from build123d import *

# Parameters (mm, degrees)
ESQUISSE1_W                       = 180
ESQUISSE1_H                       = 330
BOSS_EXTRU_1_DEPTH                = 6
ESQUISSE2_R                       = 2
ESQUISSE2_R_2                     = 10
ESQUISSE2_R_3                     = 1.4
ESQUISSE2_W                       = 55
ESQUISSE2_H                       = 8
ESQUISSE2_H_2                     = 44
ENL_V_MAT_BLOC_MOTEUR_BILLE_DEPTH = 376.946804748
ESQUISSE3_W                       = 6
ESQUISSE3_H                       = 25
ESQUISSE3_W_2                     = 10
ESQUISSE3_H_2                     = 6
ESQUISSE3_W_3                     = 30
ESQUISSE3_H_3                     = 40
ENL_V_MAT_ENCOCHE_DEPTH           = 376.946804748


with BuildPart() as part:
    # Esquisse1 → Boss.-Extru.1 (new body)
    with BuildSketch(Plane.XY):
        with Locations((-90, 165)):
            Rectangle(ESQUISSE1_W, ESQUISSE1_H)
    extrude(amount=BOSS_EXTRU_1_DEPTH)

    # Esquisse2 → Enlèv. mat bloc moteur + bille (cut, through all)
    with BuildSketch(Plane.XY.offset(6)):
        with Locations((-176, 326)):
            Circle(ESQUISSE2_R)
        with Locations((-160, 305)):
            Circle(ESQUISSE2_R_2)
        with Locations((-160, 290.27)):
            Circle(ESQUISSE2_R_3)
        with Locations((-160, 275.27)):
            Circle(ESQUISSE2_R_3)
        with Locations(Location((-160, 54.73, 0), (0, 0, 180))):
            Circle(ESQUISSE2_R_3)
        with Locations(Location((-160, 39.73, 0), (0, 0, 180))):
            Circle(ESQUISSE2_R_3)
        with Locations(Location((-160, 25, 0), (0, 0, 180))):
            Circle(ESQUISSE2_R_2)
        with Locations(Location((-176, 4, 0), (0, 0, 180))):
            Circle(ESQUISSE2_R)
        with Locations((-111.5, 319)):
            Rectangle(ESQUISSE2_W, ESQUISSE2_H)
        with Locations((-111.5, 273)):
            Rectangle(ESQUISSE2_W, ESQUISSE2_H_2)
        with Locations((-111.5, 11)):
            Rectangle(ESQUISSE2_W, ESQUISSE2_H)
        with Locations((-111.5, 57)):
            Rectangle(ESQUISSE2_W, ESQUISSE2_H_2)
    extrude(amount=-ENL_V_MAT_BLOC_MOTEUR_BILLE_DEPTH, mode=Mode.SUBTRACT)

    # Esquisse3 → Enlèv. mat encoche (cut, through all)
    with BuildSketch(Plane.XY.offset(6)):
        with Locations((-3, 317.5)):
            Rectangle(ESQUISSE3_W, ESQUISSE3_H)
        with Locations((-155, 3)):
            Rectangle(ESQUISSE3_W_2, ESQUISSE3_H_2)
        with Locations((-45, 3)):
            Rectangle(ESQUISSE3_W_3, ESQUISSE3_H_2)
        with Locations((-177, 165)):
            Rectangle(ESQUISSE3_W, ESQUISSE3_H_3)
        with Locations((-177, 85)):
            Rectangle(ESQUISSE3_W, ESQUISSE3_H_3)
        with Locations((-155, 327)):
            Rectangle(ESQUISSE3_W_2, ESQUISSE3_H_2)
        with Locations((-45, 327)):
            Rectangle(ESQUISSE3_W_3, ESQUISSE3_H_2)
        with Locations((-177, 245)):
            Rectangle(ESQUISSE3_W, ESQUISSE3_H_3)
        with Locations((-3, 235)):
            Rectangle(ESQUISSE3_W, ESQUISSE3_H_3)
        with Locations((-3, 165)):
            Rectangle(ESQUISSE3_W, ESQUISSE3_H_3)
        with Locations((-3, 95)):
            Rectangle(ESQUISSE3_W, ESQUISSE3_H_3)
        with Locations((-3, 12.5)):
            Rectangle(ESQUISSE3_W, ESQUISSE3_H)
    extrude(amount=-ENL_V_MAT_ENCOCHE_DEPTH, mode=Mode.SUBTRACT)


solid = part.part
Geometry check sheet. Reference: the model listing, model coordinates, mm. A direction names the side the tool comes from. Round coordinates to 2 decimals unless told otherwise and drop trailing zeros. Order: outer loops, then holes, each group sorted by start corner. A loop starts at its lowest first (then second) coordinate and runs counter-clockwise, first axis right, second up. Notation, with made-up numbers: M 18,49 L 69,49 A12 cw 69,63 Z; hole C -15.5,3 d2. An arc over 180 degrees is marked long. Answer in a Markdown table with one row per item. Add a question column.
Item 1: Sectioned sample at C-C, the plane y = 162.5. Enter the section's corners in (x, z), plus the area to 3 significant figures.
Item 2: Depth check by flat-ended pin: pin 1 Ø1.8 at (y, z) = (164.5, 3) entering from -X; pin 2 Ø1.8 at (x, z) = (-2.5, 3) entering from +Y; pin 3 Ø1.8 at (y, z) = (328.5, 3.5) entering from +X. Enter the tip coordinate at first touch or a pass-through.
Item 3: Sectioned sample at D-D, the plane z = 3.4. State how many separate pieces and enclosed holes the cut face has, plus the area to 3 significant figures.
Item 4: Sectioned sample at B-B, the plane x = -119. Enter the section's corners in (y, z).
Item 5: Draft check along Y on faces 5 (the face through (-18, 330, 3)), 6 (the face through (-177, 65, 3)), 7 (the face through (-174, 245, 3)), 8 (the face through (0, 50, 3)). Enter one of: released by +Y, released by -Y, zero draft, split by the parting line, or undercut.
Item 6: Sectioned sample at A-A, the plane y = 260.5. Enter the section's corners in (x, z), plus the area to 3 significant figures.
Item 7: Material ranges on L1, parallel to X at y = 39.73, z = 2.15; L2, parallel to Y at x = -102, z = 5.35; L3, parallel to Y at x = -176, z = 4.4, recorded low to high. Write a range as [from, to].
Item 8: Set-up check for faces 1 (the face through (-139, 319, 3)), 2 (the face through (-45, 6, 3)), 3 (the face through (-174, 165, 3)), 4 (the face through (-6, 12, 3)): record each of +Z, -Z, +X, -X, +Y, -Y from which the full face is reachable in a straight line by a thin tool's end or side.
Filled in:
| question | item | result |
|---|---|---|
| 1 | outline | M -174,0 L -6,0 L -6,6 L -174,6 Z |
| 1 | area | 1,010 mm² |
| 2 | pin 1 | stops at x = -174 |
| 2 | pin 2 | stops at y = 305 |
| 2 | pin 3 | stops at x = -6 |
| 3 | separate pieces | 1 |
| 3 | enclosed holes | 12 |
| 3 | area | 50,800 mm² |
| 4 | outline | M 0,0 L 7,0 L 7,6 L 0,6 Z; M 15,0 L 35,0 L 35,6 L 15,6 Z; M 79,0 L 251,0 L 251,6 L 79,6 Z; M 295,0 L 315,0 L 315,6 L 295,6 Z; M 323,0 L 330,0 L 330,6 L 323,6 Z |
| 5 | face 5 | released by +Y |
| 5 | face 6 | undercut |
| 5 | face 7 | undercut |
| 5 | face 8 | zero draft |
| 6 | outline | M -174,0 L -139,0 L -139,6 L -174,6 Z; M -84,0 L 0,0 L 0,6 L -84,6 Z |
| 6 | area | 714 mm² |
| 7 | L1 | x = [-180, -161.4], [-158.6, -139], [-84, 0] |
| 7 | L2 | y = [0, 7], [15, 35], [79, 251], [295, 315], [323, 330] |
| 7 | L3 | y = [0, 2], [6, 65], [105, 145], [185, 225], [265, 324], [328, 330] |
| 8 | face 1 | +Z, -Z |
| 8 | face 2 | +Z, -Z, -Y |
| 8 | face 3 | +Z, -Z, -X |
| 8 | face 4 | +Z, -Z, +X, -Y |
